Study the drawing (mm; zero at the part's minimum x, y, z) and answer. A direction names the side the tool comes from. Coordinates: 2 decimals unless noted, no trailing zeros. Loops run counter-clockwise (first coordinate to the right, second up) from the corner with the lowest first, then second, coordinate; pieces in that order, holes last. Notation, with made-up numbers: (-39, 60.25) - (-9, 60.25) arc R18 ccw to (-9, 70.25) - close; hole circle Ø3 at (-23, 59). An arc over 180 degrees is marked (long way). Use one line per item in the form item = value. Start each with the question number.
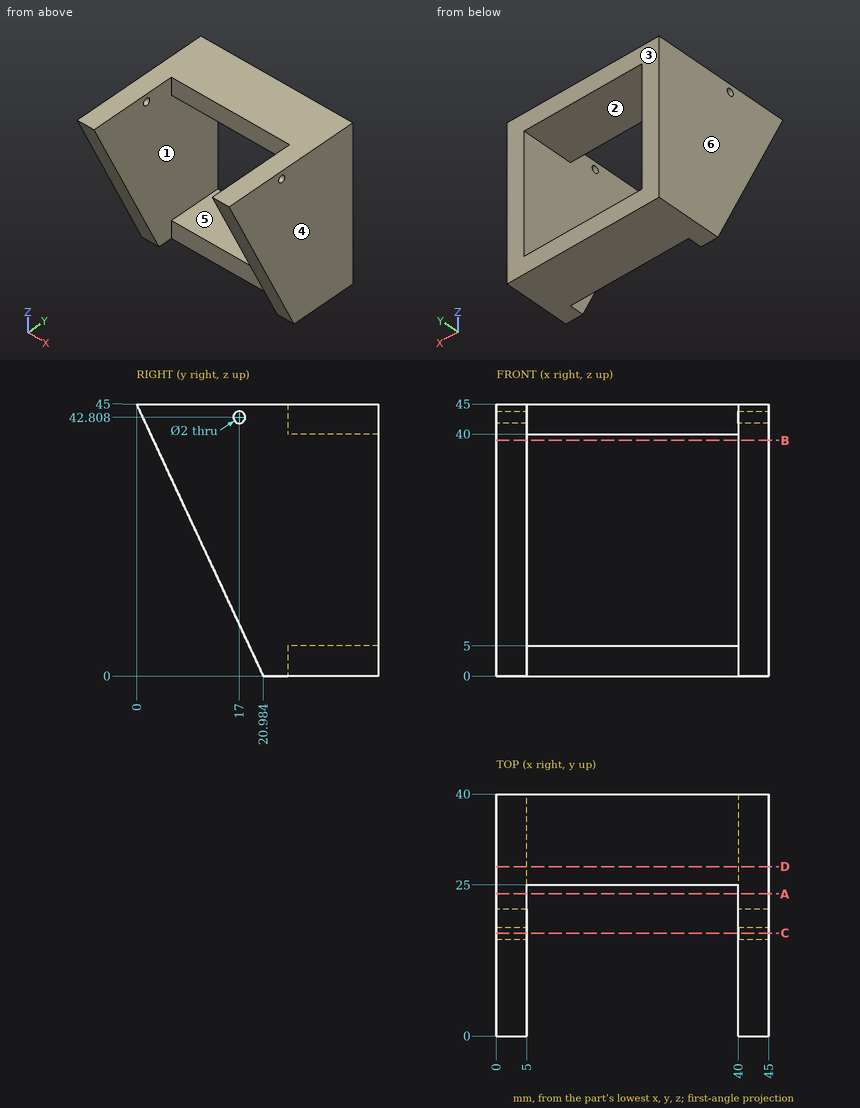
(1) For the marked faces 1, 2 and 3, determine the directions among +Z, -Z, +X, -X, +Y, -Y from which every point of the face is accessible in a straight line to the end or side of a thin tool.
(2) A cutting plane is placed at D-D (y = 28). Determine the outline of the cut face in (x, z).
(3) A cutting plane is placed at B-B (z = 39). Determine the outline of the cut face in (x, y).
(4) Determine the mould class of the marked faces 4, 5 and 6 for opening direction X: +X half, -X half, draft (parallel to the pull), parting line (faces both ways), or undercut.
(5) A cutting plane is placed at A-A (y = 23.5). Determine the outline of the cut face in (x, z).
(6) Find the intervals of material crossed by probe 1 along X at (y, z) = (22, 36.5); probe 2 along Y at (x, z) = (23, 2.5), in increasing order. Write a range as from..to.
(7) This flat-tipped pin is pushed along its axis until it touches: pin 1 Ø10 at (x, z) = (15.5, 4.5) entering from -Y. Where does it stop, or does it pass through?
(8) A cutting plane is placed at C-C (y = 17). Determine the outline of the cut face in (x, z).
Evaluation:
q1.face_1 = -Y
q1.face_2 = +Y, -Y
q1.face_3 = +Z, -Z, +X, -X, +Y
q2.outline = (0, 0) - (45, 0) - (45, 45) - (0, 45) - close; hole (5, 5) - (40, 5) - (40, 40) - (5, 40) - close
q3.outline = (0, 2.8) - (5, 2.8) - (5, 40) - (0, 40) - close; (40, 2.8) - (45, 2.8) - (45, 40) - (40, 40) - close
q4.face_4 = +X half
q4.face_5 = undercut
q4.face_6 = -X half
q5.outline = (0, 0) - (5, 0) - (5, 45) - (0, 45) - close; (40, 0) - (45, 0) - (45, 45) - (40, 45) - close
q6.probe_1 = 0..5, 40..45
q6.probe_2 = 25..40
q7.pin_1 = 25
q8.outline = (0, 8.54) - (5, 8.54) - (5, 41.81) - (0, 41.81) - close; (0, 43.81) - (5, 43.81) - (5, 45) - (0, 45) - close; (40, 8.54) - (45, 8.54) - (45, 41.81) - (40, 41.81) - close; (40, 43.81) - (45, 43.81) - (45, 45) - (40, 45) - close
